```python
from build123d import *

# Parameters (mm, degrees)
SKETCH1_R           = 60
BOSS_EXTRUDE1_DEPTH = 5
SKETCH3_W           = 14
SKETCH3_H           = 7
BOSS_EXTRUDE2_DEPTH = 5
SKETCH4_R           = 3.25
CUT_EXTRUDE1_DEPTH  = 9
SKETCH7_R           = 1.75
CUT_EXTRUDE2_DEPTH  = 5
FILLET1_R           = 10


with BuildPart() as part:
    # Sketch1 → Boss-Extrude1 (new body)
    with BuildSketch(Plane(origin=(0, 0, 0), x_dir=(1, 0, 0), z_dir=(0, 1, 0))):
        with Locations(Location((0, 0, 0), (0, 0, 270))):
            Circle(SKETCH1_R)
    extrude(amount=BOSS_EXTRUDE1_DEPTH)

    # Sketch3 → Boss-Extrude2 (add)
    with BuildSketch(Plane.XZ):
        Rectangle(SKETCH3_W, SKETCH3_H)
    extrude(amount=BOSS_EXTRUDE2_DEPTH)

    # Sketch4 → Cut-Extrude1 (cut)
    with BuildSketch(Plane(origin=(0, 5, 0), x_dir=(1, 0, 0), z_dir=(0, 1, 0))):
        with Locations((3, 0)):
            Circle(SKETCH4_R)
        with Locations((-3, 0)):
            Circle(SKETCH4_R)
    extrude(amount=-CUT_EXTRUDE1_DEPTH, mode=Mode.SUBTRACT)

    # Sketch7 → Cut-Extrude2 (cut)
    with BuildSketch(Plane(origin=(0, -4, 0), x_dir=(1, 0, 0), z_dir=(0, 1, 0))):
        with Locations(Location((-3, 0, 0), (0, 0, 270))):
            Circle(SKETCH7_R)
        with Locations(Location((3, 0, 0), (0, 0, 270))):
            Circle(SKETCH7_R)
    extrude(amount=-CUT_EXTRUDE2_DEPTH, mode=Mode.SUBTRACT)

    # Fillet1
    # the kernel refuses this fillet: 10 mm, written as the material it adds along each edge
    with BuildSketch(Plane(origin=(7, 0, 3.5), x_dir=(0, 0, 1), z_dir=(-1, 0, 0)), Plane(origin=(-7, 0, -3.5), x_dir=(0, 0, -1), z_dir=(1, 0, 0))) as fillet1_piece_1:
        with BuildLine():
            CenterArc((8.660254038, -10), FILLET1_R, 90, 60)
            Line((0, -5), (-0.173205081, -4.9))
            ThreePointArc((-0.173205081, -4.9), (-0.2, -2.5), (-0.2, 0))
            Line((-0.2, 0), (0, 0.2))
            Line((0, 0.2), (8.660254038, 0.2))
            Line((8.660254038, 0.2), (8.660254038, 0))
        make_face()
    extrude(amount=14)
    with BuildSketch(Plane(origin=(7, 0, -3.5), x_dir=(1, 0, 0), z_dir=(0, 0, 1)), Plane(origin=(-7, 0, 3.5), x_dir=(-1, 0, 0), z_dir=(0, 0, -1))) as fillet1_piece_2:
        with BuildLine():
            CenterArc((8.660254038, -10), FILLET1_R, 90, 60)
            Line((0, -5), (-0.173205081, -4.9))
            ThreePointArc((-0.173205081, -4.9), (-0.2, -2.5), (-0.2, 0))
            Line((-0.2, 0), (0, 0.2))
            Line((0, 0.2), (8.660254038, 0.2))
            Line((8.660254038, 0.2), (8.660254038, 0))
        make_face()
    extrude(amount=7)
    with BuildSketch(Plane(origin=(28.650635095, 0, 3.5), x_dir=(0, 0, 1), z_dir=(-1, 0, 0))) as fillet1_piece_3a_section:
        with BuildLine():
            CenterArc((8.660254038, -10), FILLET1_R, 90, 60)
            Line((0, -5), (-0.173205081, -4.9))
            ThreePointArc((-0.173205081, -4.9), (-0.2, -2.5), (-0.2, 0))
            Line((-0.2, 0), (0, 0.2))
            Line((0, 0.2), (8.660254038, 0.2))
            Line((8.660254038, 0.2), (8.660254038, 0))
        make_face()
    fillet1_piece_3a = extrude(amount=35.650635095, mode=Mode.PRIVATE)
    fillet1_piece_3a = split(fillet1_piece_3a, bisect_by=Plane(origin=(7, -1.295167111, 5.663104458), z_dir=(1, 0, 0)), keep=Keep.TOP, mode=Mode.PRIVATE)
    with BuildSketch(Plane(origin=(7, 0, -3.5), x_dir=(1, 0, 0), z_dir=(0, 0, 1))) as fillet1_piece_3b_section:
        with BuildLine():
            CenterArc((8.660254038, -10), FILLET1_R, 90, 60)
            Line((0, -5), (-0.173205081, -4.9))
            ThreePointArc((-0.173205081, -4.9), (-0.2, -2.5), (-0.2, 0))
            Line((-0.2, 0), (0, 0.2))
            Line((0, 0.2), (8.660254038, 0.2))
            Line((8.660254038, 0.2), (8.660254038, 0))
        make_face()
    fillet1_piece_3b = extrude(amount=28.650635095, mode=Mode.PRIVATE)
    fillet1_piece_3b = split(fillet1_piece_3b, bisect_by=Plane(origin=(9.163104458, -1.295167111, 3.5), z_dir=(0, 0, 1)), keep=Keep.TOP, mode=Mode.PRIVATE)
    fillet1_piece_3 = fillet1_piece_3a & fillet1_piece_3b
    add(fillet1_piece_3)
    with BuildSketch(Plane(origin=(-7, 0, 25.150635095), x_dir=(-1, 0, 0), z_dir=(0, 0, -1))) as fillet1_piece_4a_section:
        with BuildLine():
            CenterArc((8.660254038, -10), FILLET1_R, 90, 60)
            Line((0, -5), (-0.173205081, -4.9))
            ThreePointArc((-0.173205081, -4.9), (-0.2, -2.5), (-0.2, 0))
            Line((-0.2, 0), (0, 0.2))
            Line((0, 0.2), (8.660254038, 0.2))
            Line((8.660254038, 0.2), (8.660254038, 0))
        make_face()
    fillet1_piece_4a = extrude(amount=28.650635095, mode=Mode.PRIVATE)
    fillet1_piece_4a = split(fillet1_piece_4a, bisect_by=Plane(origin=(-9.163104458, -1.295167111, 3.5), z_dir=(0, 0, 1)), keep=Keep.TOP, mode=Mode.PRIVATE)
    with BuildSketch(Plane(origin=(7, 0, 3.5), x_dir=(0, 0, 1), z_dir=(-1, 0, 0))) as fillet1_piece_4b_section:
        with BuildLine():
            CenterArc((8.660254038, -10), FILLET1_R, 90, 60)
            Line((0, -5), (-0.173205081, -4.9))
            ThreePointArc((-0.173205081, -4.9), (-0.2, -2.5), (-0.2, 0))
            Line((-0.2, 0), (0, 0.2))
            Line((0, 0.2), (8.660254038, 0.2))
            Line((8.660254038, 0.2), (8.660254038, 0))
        make_face()
    fillet1_piece_4b = extrude(amount=35.650635095, mode=Mode.PRIVATE)
    fillet1_piece_4b = split(fillet1_piece_4b, bisect_by=Plane(origin=(-7, -1.295167111, 5.663104458), z_dir=(-1, 0, 0)), keep=Keep.TOP, mode=Mode.PRIVATE)
    fillet1_piece_4 = fillet1_piece_4a & fillet1_piece_4b
    add(fillet1_piece_4)
    with BuildSketch(Plane(origin=(7, 0, -25.150635095), x_dir=(1, 0, 0), z_dir=(0, 0, 1))) as fillet1_piece_5a_section:
        with BuildLine():
            CenterArc((8.660254038, -10), FILLET1_R, 90, 60)
            Line((0, -5), (-0.173205081, -4.9))
            ThreePointArc((-0.173205081, -4.9), (-0.2, -2.5), (-0.2, 0))
            Line((-0.2, 0), (0, 0.2))
            Line((0, 0.2), (8.660254038, 0.2))
            Line((8.660254038, 0.2), (8.660254038, 0))
        make_face()
    fillet1_piece_5a = extrude(amount=28.650635095, mode=Mode.PRIVATE)
    fillet1_piece_5a = split(fillet1_piece_5a, bisect_by=Plane(origin=(9.163104458, -1.295167111, -3.5), z_dir=(0, 0, -1)), keep=Keep.TOP, mode=Mode.PRIVATE)
    with BuildSketch(Plane(origin=(-7, 0, -3.5), x_dir=(0, 0, -1), z_dir=(1, 0, 0))) as fillet1_piece_5b_section:
        with BuildLine():
            CenterArc((8.660254038, -10), FILLET1_R, 90, 60)
            Line((0, -5), (-0.173205081, -4.9))
            ThreePointArc((-0.173205081, -4.9), (-0.2, -2.5), (-0.2, 0))
            Line((-0.2, 0), (0, 0.2))
            Line((0, 0.2), (8.660254038, 0.2))
            Line((8.660254038, 0.2), (8.660254038, 0))
        make_face()
    fillet1_piece_5b = extrude(amount=35.650635095, mode=Mode.PRIVATE)
    fillet1_piece_5b = split(fillet1_piece_5b, bisect_by=Plane(origin=(7, -1.295167111, -5.663104458), z_dir=(1, 0, 0)), keep=Keep.TOP, mode=Mode.PRIVATE)
    fillet1_piece_5 = fillet1_piece_5a & fillet1_piece_5b
    add(fillet1_piece_5)
    with BuildSketch(Plane(origin=(-7, 0, 3.5), x_dir=(-1, 0, 0), z_dir=(0, 0, -1))) as fillet1_piece_6a_section:
        with BuildLine():
            CenterArc((8.660254038, -10), FILLET1_R, 90, 60)
            Line((0, -5), (-0.173205081, -4.9))
            ThreePointArc((-0.173205081, -4.9), (-0.2, -2.5), (-0.2, 0))
            Line((-0.2, 0), (0, 0.2))
            Line((0, 0.2), (8.660254038, 0.2))
            Line((8.660254038, 0.2), (8.660254038, 0))
        make_face()
    fillet1_piece_6a = extrude(amount=28.650635095, mode=Mode.PRIVATE)
    fillet1_piece_6a = split(fillet1_piece_6a, bisect_by=Plane(origin=(-9.163104458, -1.295167111, -3.5), z_dir=(0, 0, -1)), keep=Keep.TOP, mode=Mode.PRIVATE)
    with BuildSketch(Plane(origin=(-28.650635095, 0, -3.5), x_dir=(0, 0, -1), z_dir=(1, 0, 0))) as fillet1_piece_6b_section:
        with BuildLine():
            CenterArc((8.660254038, -10), FILLET1_R, 90, 60)
            Line((0, -5), (-0.173205081, -4.9))
            ThreePointArc((-0.173205081, -4.9), (-0.2, -2.5), (-0.2, 0))
            Line((-0.2, 0), (0, 0.2))
            Line((0, 0.2), (8.660254038, 0.2))
            Line((8.660254038, 0.2), (8.660254038, 0))
        make_face()
    fillet1_piece_6b = extrude(amount=35.650635095, mode=Mode.PRIVATE)
    fillet1_piece_6b = split(fillet1_piece_6b, bisect_by=Plane(origin=(-7, -1.295167111, -5.663104458), z_dir=(-1, 0, 0)), keep=Keep.TOP, mode=Mode.PRIVATE)
    fillet1_piece_6 = fillet1_piece_6a & fillet1_piece_6b
    add(fillet1_piece_6)


solid = part.part
```
The model under review builds one solid part; all positions refer to its coordinate system, in mm. A direction names the side the tool comes from. Give positions to 0.01 mm unless a question says otherwise; leave off trailing zeros. Order: outer loops, then holes, each group sorted by start corner. A loop starts at its lowest first (then second) coordinate and runs counter-clockwise, first axis right, second up. Notation, with made-up numbers: (25, -9) - (54, -9) arc R15 cw to (54, -4) - close; hole circle Ø4 at (44.5, 42.25). An arc over 180 degrees is marked (long way). Use CSV: the item, a comma, the result in double quotes. Start each with the question number.
Q1. We need section B-B, the plane y = 1.75. Write out the cut boundary in (x, z).
Q2. Tool access review of faces 5 (the cylindrical face through (1.29, -4.49, -0.38)), 6 (the cylindrical face through (-6.248, 0.563, -0.125)): name each direction out of +Z, -Z, +X, -X, +Y, -Y from which nothing blocks a thin tool from reaching the whole face with its end or side.
Q3. The part is to be moulded in two halves that separate along Z. For faces 1 (the flat face through (0, -4, 0)), 2 (the cylindrical face through (0.219, -0.789, 8.267)), 3 (the cylindrical face through (2.64, 2.46, -59.94)), 4 (the cylindrical face through (11.767, -0.789, -0.17)), say which applies: +Z half, -Z half, draft (parallel to the pull), parting line (faces both ways), or undercut.
Q4. We need section A-A, the plane x = 3. Write out the cut boundary in (y, z), and give its area (3 significant figures).
Q5. We need section D-D, the plane z = 7.5. Write out the cut boundary in (x, y), and give its area (3 significant figures).
Q6. We need section C-C, the plane x = -11. Write out the cut boundary in (y, z), and give its area (3 significant figures).
Q7. To check wall thickness, follow line 1 along X through (y, z) = (-4.55, 0); line 2 along Y through (x, z) = (-34, 45); line 3 along Z through (x, y) = (3, 2). State the ranges of each line that lie inside material, in increasing order. Write a range as [from, to].
Q8. Clearance check with flat-ended pins moving along their axes: pin 1 Ø3 at (x, y) = (29, 1) entering from -Z; pin 2 Ø1.5 at (x, y) = (-37, 4) entering from +Z; pin 3 Ø2 at (x, z) = (-1, 0) entering from +Y. State where each tip first meets the part, or that it passes through.
Outcome:
1,outline,"circle Ø120 at (0, 0); hole (0, -1.25) arc R3.25 ccw (long way) to (0, 1.25) arc R3.25 ccw (long way) to start"
2,face 5,"+Y, -Y"
2,face 6,"+Y"
3,face 1,"undercut"
3,face 2,"+Z half"
3,face 3,"parting line"
3,face 4,"draft"
4,outline,"(-5, -3.5) arc R10 cw to (0, -12.16) - (0, -59.92) - (5, -59.92) - (5, -3.25) - (-4, -3.25) - (-4, -1.75) - (-5, -1.75) - close; (-5, 1.75) - (-4, 1.75) - (-4, 3.25) - (5, 3.25) - (5, 59.92) - (0, 59.92) - (0, 12.16) arc R10 cw to (-5, 3.5) - close"
4,area,"597 mm^2"
5,outline,"(-59.53, 0) - (-15.66, 0) arc R10 cw to (-11, -1.15) - (11, -1.15) arc R10 cw to (15.66, 0) - (59.53, 0) - (59.53, 5) - (-59.53, 5) - close"
5,area,"624 mm^2"
6,outline,"(-1.15, -7.5) arc R10 cw to (0, -12.16) - (0, -58.98) - (5, -58.98) - (5, 58.98) - (0, 58.98) - (0, 12.16) arc R10 cw to (-1.15, 7.5) - close"
6,area,"611 mm^2"
7,line 1,"x = [-7.28, -4.75], [-1.25, 1.25], [4.75, 7.28]"
7,line 2,"y = [0, 5]"
7,line 3,"z = [-59.92, -3.25], [3.25, 59.92]"
8,pin 1,"stops at z = -53.33"
8,pin 2,"stops at z = 47.81"
8,pin 3,"stops at y = -4"
